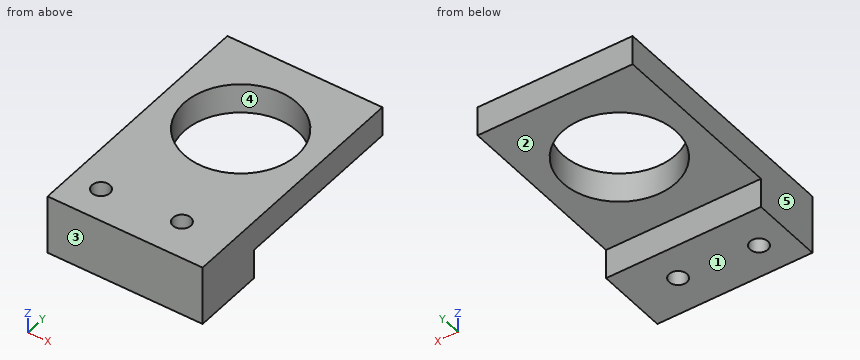
from build123d import *

# Parameters (mm, degrees)
CROQUIS1_W              = 26
CROQUIS1_H              = 42
CROQUIS1_R              = 9.5
CROQUIS1_R_2            = 1.5
SALIENTE_EXTRUIR1_DEPTH = 10
CROQUIS2_W              = 5
CROQUIS2_H              = 30
CORTAR_EXTRUIR1_DEPTH   = 40


with BuildPart() as part:
    # Croquis1 → Saliente-Extruir1 (new body)
    with BuildSketch(Plane.XY):
        with Locations((0, -6)):
            Rectangle(CROQUIS1_W, CROQUIS1_H)
        Circle(CROQUIS1_R, mode=Mode.SUBTRACT)
        with Locations((-8, -21.5)):
            Circle(CROQUIS1_R_2, mode=Mode.SUBTRACT)
        with Locations((5, -20.7)):
            Circle(CROQUIS1_R_2, mode=Mode.SUBTRACT)
    extrude(amount=SALIENTE_EXTRUIR1_DEPTH)

    # Croquis2 → Cortar-Extruir1 (cut)
    with BuildSketch(Plane.ZY.offset(13)):
        with Locations((2.5, 0)):
            Rectangle(CROQUIS2_W, CROQUIS2_H)
    extrude(amount=-CORTAR_EXTRUIR1_DEPTH, mode=Mode.SUBTRACT)


solid = part.part
The listing builds one solid part. Answer for the finished solid, in the listing's coordinates (mm). Face numbers are marked on the shaded views. A direction names the side the tool comes from. Coordinates: 2 decimals unless noted, no trailing zeros. Loops run counter-clockwise (first coordinate to the right, second up) from the corner with the lowest first, then second, coordinate; pieces in that order, holes last. Notation, with made-up numbers: (61, -20.75) -> (107, -20.75) arc R19 ccw to (107, 14.25) -> close; hole circle Ø3 at (40.5, -27). An arc over 180 degrees is marked (long way). Answer in a Markdown table with one row per item. Add a question column.
1. The part is cut by section D-D, the plane x = 5.5. Write down the section's boundary in (y, z).
2. The part is cut by section A-A, the plane y = 0. Write down the section's boundary in (x, z).
3. The part is cut by section C-C, the plane z = 1.25. Write down the section's boundary in (x, y).
4. The part is cut by section B-B, the plane x = 0. Write down the section's boundary in (y, z).
5. Flat-ended cylindrical pins translate along their axes: P1, Ø1, axis at x = -1.5, y = -11.5, coming from the -Z side; P2, Ø4, axis at x = -1.5, z = 2, coming from the +Y side; P3, Ø4, axis at x = -8, y = -21.5, coming from the -Z side. Find the tip coordinate at first contact, or state that the pin passes through.
6. Consider line 1 (Y direction, x = 0, z = 7.05); line 2 (X direction, y = 0, z = 8.2); line 3 (Y direction, x = -8, z = 7.5). Determine where each line is inside the solid, lowest interval first. Write a range as [from, to].
7. Determine the mould class of the marked faces 3, 4 and 5 for opening direction Y: +Y half, -Y half, draft (parallel to the pull), parting line (faces both ways), or undercut.
8. For the marked faces 1 and 2, determine the directions among +Z, -Z, +X, -X, +Y, -Y from which every point of the face is accessible in a straight line to the end or side of a thin tool.
Answer below:
| question | item | result |
|---|---|---|
| 1 | outline | (-27, 0) -> (-22.11, 0) -> (-22.11, 10) -> (-27, 10) -> close; (-19.29, 0) -> (-15, 0) -> (-15, 5) -> (-7.75, 5) -> (-7.75, 10) -> (-19.29, 10) -> close; (7.75, 5) -> (15, 5) -> (15, 10) -> (7.75, 10) -> close |
| 2 | outline | (-13, 5) -> (-9.5, 5) -> (-9.5, 10) -> (-13, 10) -> close; (9.5, 5) -> (13, 5) -> (13, 10) -> (9.5, 10) -> close |
| 3 | outline | (-13, -27) -> (13, -27) -> (13, -15) -> (-13, -15) -> close; hole circle Ø3 at (-8, -21.5); hole circle Ø3 at (5, -20.7) |
| 4 | outline | (-27, 0) -> (-15, 0) -> (-15, 5) -> (-9.5, 5) -> (-9.5, 10) -> (-27, 10) -> close; (9.5, 5) -> (15, 5) -> (15, 10) -> (9.5, 10) -> close |
| 5 | P1 | z = 5 |
| 5 | P2 | y = -15 |
| 5 | P3 | z = 0 |
| 6 | line 1 | [-27, -9.5], [9.5, 15] |
| 6 | line 2 | [-13, -9.5], [9.5, 13] |
| 6 | line 3 | [-27, -23], [-20, -5.12], [5.12, 15] |
| 7 | face 3 | -Y half |
| 7 | face 4 | undercut |
| 7 | face 5 | draft |
| 8 | face 1 | -Z, +X, -X, +Y, -Y |
| 8 | face 2 | -Z, +X, -X, +Y |
